```python
from build123d import *

# Parameters (mm, degrees)
F0_W     = 123.999998
F0_H     = 229.999998
F0_W_2   = 119.999998
F0_H_2   = 225.999998
F1_DEPTH = 25
F0_R     = 2
F0_W_3   = 20
F0_H_3   = 55
F0_H_4   = 23
F2_DEPTH = 2
F4_W     = 11
F4_H     = 74.715774
F5_DEPTH = 150


with BuildPart() as f1:
    # F0 (on Top) → F1 (new body)
    with BuildSketch(Plane.XY):
        Rectangle(F0_W, F0_H)
        Rectangle(F0_W_2, F0_H_2, mode=Mode.SUBTRACT)
    extrude(amount=-F1_DEPTH)

    # F0 (on Top) → F2 (join)
    with BuildSketch(Plane.XY):
        Rectangle(F0_W_2, F0_H_2)
        with Locations((-47.997308, -66.012282)):
            Circle(F0_R, mode=Mode.SUBTRACT)
        with Locations((-43.749999, -84.15)):
            Circle(F0_R, mode=Mode.SUBTRACT)
        with Locations((-22.75, -84.15)):
            Circle(F0_R, mode=Mode.SUBTRACT)
        with Locations((-47.997308, -44.012282)):
            Circle(F0_R, mode=Mode.SUBTRACT)
        with Locations((-47.997308, -22.012282)):
            Circle(F0_R, mode=Mode.SUBTRACT)
        with Locations((-47.997308, -0.012282)):
            Circle(F0_R, mode=Mode.SUBTRACT)
        with Locations((-23.997308, -0.012282)):
            Circle(F0_R, mode=Mode.SUBTRACT)
        with Locations((1.25, -84.15)):
            Circle(F0_R, mode=Mode.SUBTRACT)
        with Locations((25.25, -84.15)):
            Circle(F0_R, mode=Mode.SUBTRACT)
        with Locations((24.002692, -66.012282)):
            Circle(F0_R, mode=Mode.SUBTRACT)
        with Locations((49.750001, -84.15)):
            Circle(F0_R, mode=Mode.SUBTRACT)
        with Locations((48.002692, -66.012282)):
            Circle(F0_R, mode=Mode.SUBTRACT)
        with Locations((2.25, -51.15)):
            Rectangle(F0_W_3, F0_H_3, mode=Mode.SUBTRACT)
        with Locations((24.002692, -44.012282)):
            Circle(F0_R, mode=Mode.SUBTRACT)
        with Locations((0.002692, -0.012282)):
            Circle(F0_R, mode=Mode.SUBTRACT)
        with Locations((24.002692, -22.012282)):
            Circle(F0_R, mode=Mode.SUBTRACT)
        with Locations((24.002692, -0.012282)):
            Circle(F0_R, mode=Mode.SUBTRACT)
        with Locations((48.002692, -44.012282)):
            Circle(F0_R, mode=Mode.SUBTRACT)
        with Locations((48.002692, -22.012282)):
            Circle(F0_R, mode=Mode.SUBTRACT)
        with Locations((48.002692, -0.012282)):
            Circle(F0_R, mode=Mode.SUBTRACT)
        with Locations((-47.997308, 21.987718)):
            Circle(F0_R, mode=Mode.SUBTRACT)
        with Locations((-47.997308, 43.987718)):
            Circle(F0_R, mode=Mode.SUBTRACT)
        with Locations((-23.997308, 21.987718)):
            Circle(F0_R, mode=Mode.SUBTRACT)
        with Locations((-23.997308, 43.987718)):
            Circle(F0_R, mode=Mode.SUBTRACT)
        with Locations((-43.749999, 84.15)):
            Circle(F0_R, mode=Mode.SUBTRACT)
        with Locations((-22.75, 84.15)):
            Circle(F0_R, mode=Mode.SUBTRACT)
        with Locations((-10.3, 66)):
            Rectangle(F0_W_3, F0_H_4, mode=Mode.SUBTRACT)
        with Locations((0.002692, 21.987718)):
            Circle(F0_R, mode=Mode.SUBTRACT)
        with Locations((24.002692, 21.987718)):
            Circle(F0_R, mode=Mode.SUBTRACT)
        with Locations((0.002692, 43.987718)):
            Circle(F0_R, mode=Mode.SUBTRACT)
        with Locations((24.002692, 43.987718)):
            Circle(F0_R, mode=Mode.SUBTRACT)
        with Locations((48.002692, 21.987718)):
            Circle(F0_R, mode=Mode.SUBTRACT)
        with Locations((48.002692, 43.987718)):
            Circle(F0_R, mode=Mode.SUBTRACT)
        with Locations((1.25, 84.15)):
            Circle(F0_R, mode=Mode.SUBTRACT)
        with Locations((24.002692, 65.987718)):
            Circle(F0_R, mode=Mode.SUBTRACT)
        with Locations((25.25, 84.15)):
            Circle(F0_R, mode=Mode.SUBTRACT)
        with Locations((48.002692, 65.987718)):
            Circle(F0_R, mode=Mode.SUBTRACT)
        with Locations((49.750001, 84.15)):
            Circle(F0_R, mode=Mode.SUBTRACT)
    extrude(amount=-F2_DEPTH)

    # F4 (on face) → F5 (cut)
    with BuildSketch(Plane.YZ.offset(61.999999)):
        Polygon((114.999999, -88.085778), (114.999999, 20.739374), (103.999999, 20.739374), (103.999999, -53.001843), (103.999999, -88.085778), align=None)
        Polygon((103.999999, -88.085778), (103.999999, -53.001843), (-103.999999, -53.001843), (-114.999999, -53.001843), (-114.999999, -88.085778), align=None)
        with Locations((-109.499999, -15.643956)):
            Rectangle(F4_W, F4_H)
    extrude(amount=-F5_DEPTH, mode=Mode.SUBTRACT)


solid = f1.part
```
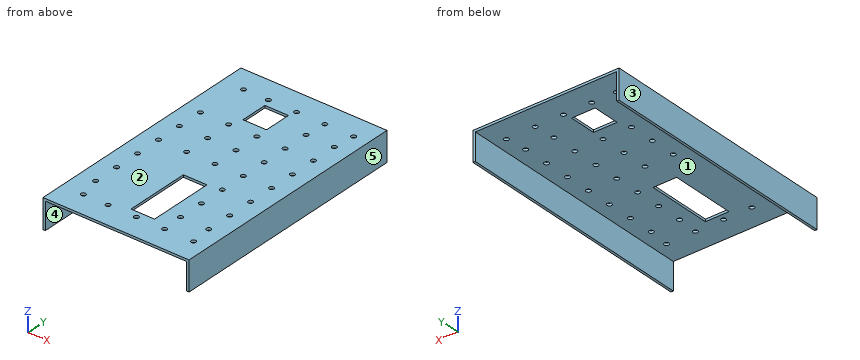
Part model, mm, in its own coordinate system. Face numbers are marked on the shaded views. A direction names the side the tool comes from. Round coordinates to 2 decimals unless told otherwise and drop trailing zeros. Order: outer loops, then holes, each group sorted by start corner. A loop starts at its lowest first (then second) coordinate and runs counter-clockwise, first axis right, second up. Notation, with made-up numbers: M -16,-37.5 L 18,-37.5 A26 cw 18,-5.5 Z; hole C 67,68 d8. An arc over 180 degrees is marked long. Answer in a Markdown table with one row per item. Add a question column.
Q1. Mould opens along X. For the marked faces 3, 4 and 5 say: +X half, -X half, draft (parallel to the pull), parting line (faces both ways), or undercut.
Q2. Cut at A-A on y = -84.15. Give the cut face in (x, z).
Q3. Pin check, flat tips, straight feed: pin 1 (4 mm diameter, centred on x = 14, y = -73.5, fed in from -Z); pin 2 (3 mm diameter, centred on x = 49.75, y = -84.15, fed in from +Z). Stop position of each tip, or through.
Q4. 3-axis set-ups, long thin cutter, end or side, ignore diameter. For the marked faces 1 and 2: which of +Z, -Z, +X, -X, +Y, -Y reach the whole face in a straight line?
Q5. Wall check: L1, parallel to Y at x = -43.75, z = -0.4; L2, parallel to X at y = 69.5, z = -2.5; L3, parallel to Y at x = 11.5, z = -1. Give the ranges that are in metal, low to high. Write a range as from..to.
Q6. Cut at D-D on x = -43.75. Give the cut face in (y, z), and give its area (3 significant figures).
Q7. Cut at C-C on z = -5.5. Give the cut face in (x, y).
Q8. Cut at B-B on x = 7. Give the cut face in (y, z), and give its area (3 significant figures).
Established:
| question | item | result |
|---|---|---|
| 1 | face 3 | -X half |
| 1 | face 4 | undercut |
| 1 | face 5 | +X half |
| 2 | outline | M -62,-25 L -60,-25 L -60,-2 L -45.75,-2 L -45.75,0 L -62,0 Z; M -41.75,-2 L -24.75,-2 L -24.75,0 L -41.75,0 Z; M -20.75,-2 L -0.75,-2 L -0.75,0 L -20.75,0 Z; M 3.25,-2 L 23.25,-2 L 23.25,0 L 3.25,0 Z; M 27.25,-2 L 47.75,-2 L 47.75,0 L 27.25,0 Z; M 51.75,-2 L 60,-2 L 60,-25 L 62,-25 L 62,0 L 51.75,0 Z |
| 3 | pin 1 | stops at z = -2 |
| 3 | pin 2 | passes through |
| 4 | face 1 | -Z, +Y, -Y |
| 4 | face 2 | +Z, +X, -X, +Y, -Y |
| 5 | L1 | y = -104..-86.15, -82.15..82.15, 86.15..104 |
| 5 | L2 | x = -62..-60, 60..62 |
| 5 | L3 | y = -104..-78.65, -23.65..104 |
| 6 | outline | M -104,-2 L -86.15,-2 L -86.15,0 L -104,0 Z; M -82.15,-2 L 82.15,-2 L 82.15,0 L -82.15,0 Z; M 86.15,-2 L 104,-2 L 104,0 L 86.15,0 Z |
| 6 | area | 400 mm2 |
| 7 | outline | M -62,-104 L -60,-104 L -60,104 L -62,104 Z; M 60,-104 L 62,-104 L 62,104 L 60,104 Z |
| 8 | outline | M -104,-2 L -78.65,-2 L -78.65,0 L -104,0 Z; M -23.65,-2 L 104,-2 L 104,0 L -23.65,0 Z |
| 8 | area | 306 mm2 |
